The model under review builds one solid part; all positions refer to its coordinate system, in mm. Face numbers are marked on the shaded views. A direction names the side the tool comes from. Give positions to 0.01 mm unless a question says otherwise; leave off trailing zeros. Loops run counter-clockwise (first coordinate to the right, second up) from the corner with the lowest first, then second, coordinate; pieces in that order, holes last. Notation, with made-up numbers: M 36,43.25 L 90,43.25 A12 ccw 90,54.25 Z; hole C 88.25,-15.75 d3. An arc over 180 degrees is marked long. Put each result on its own line as item: value. Start each with the question number.
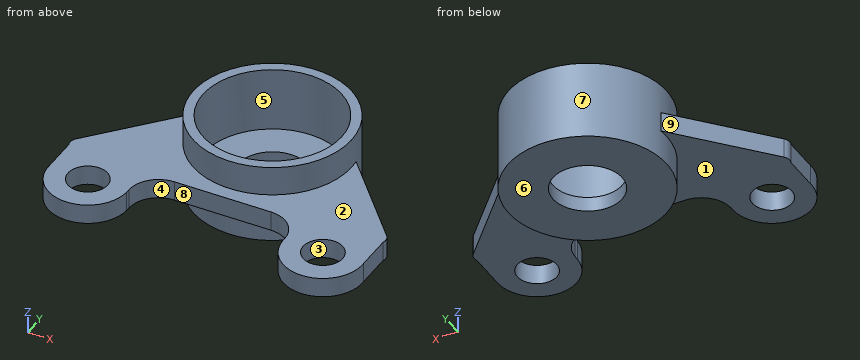
from build123d import *

# Parameters (mm, degrees)
BOSS_EXTRUDE1_DEPTH      = 4
FILLET1_R                = 8
FILLET2_R                = 2
SKETCH3_W                = 16
SKETCH3_H                = 8
BOSS_EXTRUDE2_DEPTH      = 4
SKETCH10_R               = 8
BOSS_EXTRUDE3_DEPTH      = 4
FILLET3_R                = 6
SKETCH11_R               = 4
CUT_EXTRUDE2_DEPTH       = 4
FILLET3_OF_MIRROR1_R     = 6
BOSS_EXTRUDE4_DEPTH      = 6
BOSS_EXTRUDE4_DEPTH_BACK = 10
SKETCH8_R                = 16
SKETCH13_R               = 14
CUT_EXTRUDE3_DEPTH       = 13
SKETCH17_R               = 7
CUT_EXTRUDE4_DEPTH       = 13


with BuildPart() as part:
    # Sketch2 → Boss-Extrude1 (new body)
    with BuildSketch(Plane.XY):
        Polygon((-24.718317205, 0), (44.079761222, 0), (9.680722008, 38.594041061), align=None)
    extrude(amount=BOSS_EXTRUDE1_DEPTH)

    # Fillet1
    fillet1_edges = [part.edges().sort_by_distance(p)[0] for p in [
        (9.680722008, 38.594041061, 2),
    ]]
    fillet(fillet1_edges, radius=FILLET1_R)

    # Fillet2
    fillet2_edges = [part.edges().sort_by_distance(p)[0] for p in [
        (44.079761222, 0, 2),
        (-24.718317205, 0, 2),
    ]]
    fillet(fillet2_edges, radius=FILLET2_R)

    # Sketch3 → Boss-Extrude2 (add)
    with BuildSketch(Plane.XY):
        with Locations((-14.081618267, -2.818082449)):
            Rectangle(SKETCH3_W, SKETCH3_H)
    boss_extrude2 = extrude(amount=BOSS_EXTRUDE2_DEPTH)

    # Sketch10 → Boss-Extrude3 (add)
    with BuildSketch(Plane.XY.offset(4)):
        with Locations((-14.092338513, -6.548407243)):
            Circle(SKETCH10_R)
    boss_extrude3 = extrude(amount=-BOSS_EXTRUDE3_DEPTH)

    # Fillet3
    fillet3_edges = [part.edges().sort_by_distance(p)[0] for p in [
        (-6.081618267, 0, 2),
    ]]
    fillet(fillet3_edges, radius=FILLET3_R)

    # Sketch11 → Cut-Extrude2 (cut)
    with BuildSketch(Plane.XY.offset(4)):
        with Locations((-14.092338513, -6.548407243)):
            Circle(SKETCH11_R)
    cut_extrude2 = extrude(amount=-CUT_EXTRUDE2_DEPTH, mode=Mode.SUBTRACT)

    # Mirror1: Boss-Extrude2, Boss-Extrude3, Cut-Extrude2 across plane
    add(boss_extrude2.mirror(Plane(origin=(9.7, 0, 0), x_dir=(0, 0, 1), z_dir=(1, 0, 0))))
    add(boss_extrude3.mirror(Plane(origin=(9.7, 0, 0), x_dir=(0, 0, 1), z_dir=(1, 0, 0))))
    add(cut_extrude2.mirror(Plane(origin=(9.7, 0, 0), x_dir=(0, 0, 1), z_dir=(1, 0, 0))), mode=Mode.SUBTRACT)

    # Fillet3 of Mirror1
    fillet3_of_mirror1_edges = [part.edges().sort_by_distance(p)[0] for p in [
        (25.481618267, 0, 2),
    ]]
    fillet(fillet3_of_mirror1_edges, radius=FILLET3_OF_MIRROR1_R)

    # Sketch8 → Boss-Extrude4 (add, two sides: drawn at the far end of the back side and taken through both)
    with BuildSketch(Plane.XY.offset(4).offset(-BOSS_EXTRUDE4_DEPTH_BACK)):
        with Locations((9.680722008, 18.821374391)):
            Circle(SKETCH8_R)
    extrude(amount=BOSS_EXTRUDE4_DEPTH + BOSS_EXTRUDE4_DEPTH_BACK)

    # Sketch13 → Cut-Extrude3 (cut)
    with BuildSketch(Plane.XY.offset(10)):
        with Locations((9.680722008, 18.821374391)):
            Circle(SKETCH13_R)
    extrude(amount=-CUT_EXTRUDE3_DEPTH, mode=Mode.SUBTRACT)

    # Sketch17 → Cut-Extrude4 (cut)
    with BuildSketch(Plane.XY.offset(-3)):
        with Locations((9.680722008, 18.821374391)):
            Circle(SKETCH17_R)
    extrude(amount=-CUT_EXTRUDE4_DEPTH, mode=Mode.SUBTRACT)


solid = part.part
(1) We need section A-A, the plane y = 20. Write out the cut boundary in (x, z), plus the area to 3 significant figures.
(2) We need section C-C, the plane z = 1.5. State how many separate pieces and enclosed holes the cut face has, plus the area to 3 significant figures.
(3) Insertion check: pin 1 (9 mm diameter, centred on x = -14.09, y = -6.55, fed in from +Z); pin 2 (8.5 mm diameter, centred on x = 9.5, y = 16, fed in from +Z); pin 3 (4.5 mm diameter, centred on x = 5, z = 2, fed in from -Y). Each pin has a flat end and moves straight along its axis. Give the tip position at first contact, or say it passes through.
(4) Draft analysis for pull direction X (two halves, no side actions). For the marked faces 6, 7, 8 and 9, state which applies: +X half, -X half, draft (parallel to the pull), parting line (faces both ways), or undercut.
(5) We need section D-D, the plane y = -5. Write out the cut boundary in (x, z), plus the area to 3 significant figures.
(6) To check wall thickness, follow L1, parallel to Y at x = 10, z = 5.5; L2, parallel to X at y = -10, z = 2.25; L3, parallel to Z at x = -13.5, y = -1.5. State the ranges of each line that lie inside material, in increasing order. Write a range as [from, to].
(7) We need section B-B, the plane x = -15. Write out the cut boundary in (y, z).
(8) For the marked faces 1, 2, 3, 4 and 5, list the 3-axis set-ups (+Z, -Z, +X, -X, +Y, -Y) from which the entire face can be reached by the end or side of a thin tool; tool diameter is ignored.
Check sheet entries:
1. outline: M -6.89,0 L -6.28,0 L -6.28,-6 L 2.78,-6 L 2.78,-3 L -4.27,-3 L -4.27,10 L -6.28,10 L -6.28,4 L -6.89,4 Z; M 16.58,-6 L 25.64,-6 L 25.64,0 L 26.25,0 L 26.25,4 L 25.64,4 L 25.64,10 L 23.63,10 L 23.63,-3 L 16.58,-3 Z
1. area: 111 mm²
2. separate pieces: 1
2. enclosed holes: 3
2. area: 1,090 mm²
3. pin 1: stops at z = 4
3. pin 2: stops at z = -3
3. pin 3: stops at y = 0
4. face 6: draft
4. face 7: parting line
4. face 8: undercut
4. face 9: -X half
5. outline: M -22.08,0 L -17.78,0 L -17.78,4 L -22.08,4 Z; M -10.4,0 L -6,0 L -6,4 L -10.4,4 Z; M 25.4,0 L 29.8,0 L 29.8,4 L 25.4,4 Z; M 37.18,0 L 41.48,0 L 41.48,4 L 37.18,4 Z
5. area: 69.7 mm²
6. L1: y = [2.82, 4.83], [32.82, 34.82]
6. L2: x = [-21.31, -16.11], [-12.07, -6.88], [26.28, 31.47], [35.51, 40.71]
6. L3: z = [0, 4]
7. outline: M -14.5,0 L -10.44,0 L -10.44,4 L -14.5,4 Z; M -2.65,0 L 10.9,0 L 10.9,4 L -2.65,4 Z
8. face 1: -Z, -Y
8. face 2: +Z, -Y
8. face 3: +Z, -Z
8. face 4: +Z, -Z, -Y
8. face 5: +Z
